Geometry: final body of the model. Coordinates: model frame, mm. Give positions to 0.01 mm unless a question says otherwise; leave off trailing zeros. Write each loop counter-clockwise with the first axis right and the second up, starting at its lowest first coordinate (ties: lowest second). Pieces come first, ordered by that corner, then holes. Notation, with made-up numbers: (-32.75, 39.25) - (-10.75, 39.25) arc R28 ccw to (-10.75, 65.25) - close; hole circle Ø11 at (3.5, 66). An arc over 180 degrees is marked (long way). Use CSV: the item, a comma, the result in double quotes. Start each with the question number.
(1) Line query: probe 1 along Y at (x, z) = (0, 3.5); probe 2 along X at (y, z) = (5.5, 1.25); probe 3 along Y at (x, z) = (4, 5.75). Output: solid intervals per line, ascending. Write a range as [from, to].
(2) Section D-D on z = 5.75. Count the separate pieces of the cut face and the enclosed holes in it, and give its area (3 significant figures).
(3) First-contact query: pin 1 Ø2 at (x, z) = (2.5, 3.5) entering from -Y; pin 2 Ø1 at (y, z) = (-6.5, 3.5) entering from -X; pin 3 Ø2 at (x, z) = (-6.5, 8.5) entering from -Y. Flat tips, straight axial feed; report the tip coordinate or a pass-through.
(4) Draft query along Y for faces 1 (the cylindrical face through (-0.16, 8.35, 5.11)), 2 (the cylindrical face through (-1.03, -4.65, 6.26)), 3 (the flat face through (-3.338, -13.043, 6.261)), 4 (the cylindrical face through (12.034, 6.934, 6.261)). Return one class per face: released by +Y, released by -Y, zero draft, split by the parting line, or undercut.
(5) Section C-C on y = 0. Output: boundary loops of the cut face in (x, z), and give its area (3 significant figures).
(6) Section B-B on x = 0. Output: boundary loops of the cut face in (y, z).
(7) Section A-A on y = 5.25. Output: boundary loops of the cut face in (x, z), and give its area (3 significant figures).
from build123d import *

# Parameters (mm, degrees)
SKETCH1_R           = 4.7625
SKETCH1_R_2         = 1.25
BOSS_EXTRUDE1_DEPTH = 12.7
CUT_EXTRUDE1_REACH  = 27.888
SKETCH2_R           = 1.25


with BuildPart() as part:
    # Sketch1 → Boss-Extrude1 (new body)
    with BuildSketch(Plane.XY):
        with BuildLine():
            Line((-13.253372163, -1.044486042), (-7.531237528, -10.955513958))
            ThreePointArc((-7.531237528, -10.955513958), (-6.784217233, -11.816359568), (-5.770008435, -12.336431676))
            Line((-5.770008435, -12.336431676), (-0.836847118, -13.76941319))
            ThreePointArc((-0.836847118, -13.76941319), (0, -13.888495471), (0.836847118, -13.76941319))
            Line((0.836847118, -13.76941319), (5.770008435, -12.336431676))
            ThreePointArc((5.770008435, -12.336431676), (6.784217233, -11.816359568), (7.531237528, -10.955513958))
            Line((7.531237528, -10.955513958), (13.253372163, -1.044486042))
            ThreePointArc((13.253372163, -1.044486042), (13.625376182, 0.032875315), (13.568667441, 1.171241953))
            Line((13.568667441, 1.171241953), (12.343085176, 6.159975731))
            ThreePointArc((12.343085176, 6.159975731), (12.027789898, 6.944247736), (11.506238058, 7.609437458))
            Line((11.506238058, 7.609437458), (7.798659006, 11.165189723))
            ThreePointArc((7.798659006, 11.165189723), (6.841158949, 11.783484253), (5.722134635, 12))
            Line((5.722134635, 12), (-5.722134635, 12))
            ThreePointArc((-5.722134635, 12), (-6.841158949, 11.783484253), (-7.798659006, 11.165189723))
            Line((-7.798659006, 11.165189723), (-11.506238058, 7.609437458))
            ThreePointArc((-11.506238058, 7.609437458), (-12.027789898, 6.944247736), (-12.343085176, 6.159975731))
            Line((-12.343085176, 6.159975731), (-13.568667441, 1.171241953))
            ThreePointArc((-13.568667441, 1.171241953), (-13.625376182, 0.032875315), (-13.253372163, -1.044486042))
        make_face()
        Circle(SKETCH1_R, mode=Mode.SUBTRACT)
        with Locations((-8.238066653, 4.75625)):
            Circle(SKETCH1_R_2, mode=Mode.SUBTRACT)
        with Locations((8.238066653, 4.75625)):
            Circle(SKETCH1_R_2, mode=Mode.SUBTRACT)
        with Locations((0, -9.5125)):
            Circle(SKETCH1_R_2, mode=Mode.SUBTRACT)
    extrude(amount=BOSS_EXTRUDE1_DEPTH)

    # Sketch2 → Cut-Extrude1 (cut, up to next)
    with BuildSketch(Plane(origin=(0, 12, 0), x_dir=(1, 0, 0), z_dir=(0, 1, 0)), mode=Mode.PRIVATE) as cut_extrude1_sk1:
        with Locations((0, -6.35)):
            Circle(SKETCH2_R)
    cut_extrude1_tool1 = extrude(cut_extrude1_sk1.sketch, amount=-CUT_EXTRUDE1_REACH, mode=Mode.PRIVATE) & part.part
    add(cut_extrude1_tool1.solids().sort_by_distance((0, 12, 6.35))[0], mode=Mode.SUBTRACT)


solid = part.part
Check values:
1,probe 1,"y = [-13.89, -10.76], [-8.26, -4.76], [4.76, 12]"
1,probe 2,"x = [-12.51, -9.24], [-7.23, 7.23], [9.24, 12.51]"
1,probe 3,"y = [-12.85, -2.58], [2.58, 12]"
2,separate pieces,"1"
2,enclosed holes,"3"
2,area,"437 mm²"
3,pin 1,"stops at y = -13.58"
3,pin 2,"stops at x = -10.39"
3,pin 3,"stops at y = -12.41"
4,face 1,"zero draft"
4,face 2,"undercut"
4,face 3,"released by -Y"
4,face 4,"released by +Y"
5,outline,"(-13.62, 0) - (-4.76, 0) - (-4.76, 12.7) - (-13.62, 12.7) - close; (4.76, 0) - (13.62, 0) - (13.62, 12.7) - (4.76, 12.7) - close"
5,area,"225 mm²"
6,outline,"(-13.89, 0) - (-10.76, 0) - (-10.76, 12.7) - (-13.89, 12.7) - close; (-8.26, 0) - (-4.76, 0) - (-4.76, 12.7) - (-8.26, 12.7) - close; (4.76, 0) - (12, 0) - (12, 5.1) - (4.76, 5.1) - close; (4.76, 7.6) - (12, 7.6) - (12, 12.7) - (4.76, 12.7) - close"
7,outline,"(-12.57, 0) - (-9.39, 0) - (-9.39, 12.7) - (-12.57, 12.7) - close; (-7.09, 0) - (7.09, 0) - (7.09, 12.7) - (-7.09, 12.7) - close; (9.39, 0) - (12.57, 0) - (12.57, 12.7) - (9.39, 12.7) - close; hole circle Ø2.5 at (0, 6.35)"
7,area,"256 mm²"
